from build123d import *

# Parameters (mm, degrees)
BOSS_EXTRUDE1_DEPTH       = 22.5
BOSS_EXTRUDE1_DEPTH_BACK  = 22.5
SKETCH1_R                 = 3
F_6_32_TAPPED_HOLE1_D     = 2.7051
F_6_32_TAPPED_HOLE1_DEPTH = 10.35
F_6_32_TAPPED_HOLE1_TIP   = 0.81269403
FILLET1_R                 = 0.5
F_6_32_TAPPED_HOLE2_D     = 2.7051
F_6_32_TAPPED_HOLE2_DEPTH = 10.35
F_6_32_TAPPED_HOLE2_TIP   = 0.81269403


with BuildPart() as part:
    # Sketch1 → Boss-Extrude1 (new, two sides: drawn at the far end of the back side and taken through both)
    with BuildSketch(Plane(origin=(0, 0, 0), x_dir=(1, 0, 0), z_dir=(0, 1, 0)).offset(-BOSS_EXTRUDE1_DEPTH_BACK)):
        with Locations(Location((0, 0, 0), (0, 0, 270))):
            Circle(SKETCH1_R)
    extrude(amount=BOSS_EXTRUDE1_DEPTH + BOSS_EXTRUDE1_DEPTH_BACK)

    # 6-32 Tapped Hole1
    with Locations(Plane(origin=(0, 22.5, 0), x_dir=(1, 0, 0), z_dir=(0, 1, 0))):
        with Locations((0, 0)):
            Hole(F_6_32_TAPPED_HOLE1_D / 2, depth=F_6_32_TAPPED_HOLE1_DEPTH)
            with Locations((0, 0, -(F_6_32_TAPPED_HOLE1_DEPTH + F_6_32_TAPPED_HOLE1_TIP / 2))):  # 118° drill point
                Cone(0, F_6_32_TAPPED_HOLE1_D / 2, F_6_32_TAPPED_HOLE1_TIP, mode=Mode.SUBTRACT)

    # Fillet1
    fillet1_edges = [part.edges().sort_by_distance(p)[0] for p in [
        (0, -22.5, -3),
        (0, 22.5, -3),
    ]]
    fillet(fillet1_edges, radius=FILLET1_R)

    # 6-32 Tapped Hole2
    with Locations(Plane(origin=(0, -22.5, 0), x_dir=(-1, 0, 0), z_dir=(0, -1, 0))):
        with Locations((0, 0)):
            Hole(F_6_32_TAPPED_HOLE2_D / 2, depth=F_6_32_TAPPED_HOLE2_DEPTH)
            with Locations((0, 0, -(F_6_32_TAPPED_HOLE2_DEPTH + F_6_32_TAPPED_HOLE2_TIP / 2))):  # 118° drill point
                Cone(0, F_6_32_TAPPED_HOLE2_D / 2, F_6_32_TAPPED_HOLE2_TIP, mode=Mode.SUBTRACT)


solid = part.part
Here's how the part is built. I have some questions about the finished solid (model axes, mm). A direction names the side the tool comes from. Coordinates: 2 decimals unless noted, no trailing zeros. Order: outer loops, then holes, each group sorted by start corner. A loop starts at its lowest first (then second) coordinate and runs counter-clockwise, first axis right, second up. Notation, with made-up numbers: (79, 15) -> (89, 15) arc R27 cw to (89, 41) -> close; hole circle Ø4 at (-12.5, -38.75). An arc over 180 degrees is marked (long way). Answer in a Markdown table with one row per item.
(1) Will these pins go through, and if not, where does the flat tip stop? pin 1 Ø3.5 at (x, z) = (0, 0) entering from +Y; pin 2 Ø2.5 at (x, z) = (0, 0) entering from +Y; pin 3 Ø1 at (y, z) = (14, -2) entering from +X.
Answer key:
| item | result |
|---|---|
| pin 1 | y = 22.5 |
| pin 2 | y = 12.09 |
| pin 3 | x = 2.6 |
(2) Please list where these lines run through material, in increasing order: probe 1 along Y at (x, z) = (1.7, 1.95); probe 2 along X at (y, z) = (5, -0.1); probe 3 along Z at (x, y) = (1, 9).
Answer key:
| item | result |
|---|---|
| probe 1 | -22.49 to 22.49 |
| probe 2 | -3 to 3 |
| probe 3 | -2.83 to 2.83 |
(3) I want a section at B-B on y = -5. List the corners of the cut face in (x, z) for me, then the cut area to 3 significant figures.
Answer key:
| item | result |
|---|---|
| outline | circle Ø6 at (0, 0) |
| area | 28.3 mm^2 |
(4) Thinking about a two-plate mould opening in Z: for faces 3 (the face through (-1.29, 17.25, -0.41)), 4 (the face through (0.9, -0.31, 2.86)), 5 (the face through (-1.1, -22.5, 1.1)), which applies, +Z half, -Z half, draft (parallel to the pull), parting line (faces both ways), or undercut?
Answer key:
| item | result |
|---|---|
| face 3 | undercut |
| face 4 | parting line |
| face 5 | draft |
(5) On a 3-axis mill with a long thin cutter (end or side, diameter ignored), from which of +Z, -Z, +X, -X, +Y, -Y can I reach the whole of each face in a straight line? I mean faces 1 (the face through (1.29, -17.25, -0.41)), 2 (the face through (-0.05, 11.48, 0.23)). Say none if no direction works.
Answer key:
| item | result |
|---|---|
| face 1 | -Y |
| face 2 | +Y |
(6) I want a section at A-A on y = -14.5. List the corners of the cut face in (x, z) for me, then the cut area to 3 significant figures.
Answer key:
| item | result |
|---|---|
| outline | circle Ø6 at (0, 0); hole circle Ø2.71 at (0, 0) |
| area | 22.5 mm^2 |
